Here's how the part is built. I have some questions about the finished solid (model axes, mm). A direction names the side the tool comes from. Round coordinates to 2 decimals unless told otherwise and drop trailing zeros. Write each loop counter-clockwise with the first axis right and the second up, starting at its lowest first coordinate (ties: lowest second). Pieces come first, ordered by that corner, then holes. Notation, with made-up numbers: (-26, 39) - (9, 39) arc R21 ccw to (9, 43) - close; hole circle Ø3 at (45, -18). An arc over 180 degrees is marked (long way). One line per question, with ' | ' between items. Start each with the question number.
(1) For faces 5 (the flat face through (-2, -48.26, 4)), 6 (the flat face through (-2, -50.8, 3)), which set-ups out of +Z, -Z, +X, -X, +Y, -Y let a thin tool reach every point of the face, with its end or its side?
(2) Imagine slicing it at A-A (z = 3.25). Write out the boundary of the cut face in (x, y).
(3) Will these pins go through, and if not, where does the flat tip stop? pin 1 (8 mm diameter, centred on x = -18, y = -9.5, fed in from -Z); pin 2 (10 mm diameter, centred on x = 13.5, y = -35.5, fed in from +Z); pin 3 (2 mm diameter, centred on x = -8, y = -21.5, fed in from +Z).
(4) Imagine slicing it at D-D (z = -6.25). Write out the boundary of the cut face in (x, y).
(5) If I drill on L1, parallel to Y at x = -5.5, z = 9.5; L2, parallel to X at y = -32, z = 3.25; L3, parallel to X at y = -8.5, z = -9, over which ranges is the centre line in solid material (lowest first)?
(6) Thinking about a two-plate mould opening in X: for faces 1 (the flat face through (-2, -2.54, 4)), 2 (the flat face through (0, -50, 12.7)), 3 (the flat face through (-13.842, -25.044, -6.261)), 4 (the flat face through (23.497, -25, 6)), which applies, pulls with the +X half, pulls with the -X half, needs draft (parallel to the pull), parting line crosses it, or undercut?
(7) Imagine slicing it at C-C (x = -5). Write out the boundary of the cut face in (y, z), plus the area to 3 significant figures.
(8) Imagine slicing it at B-B (y = -19). Write out the boundary of the cut face in (x, z).
from build123d import *

# Parameters (mm, degrees)
F1_DEPTH = 50.8
F2_T     = -2.54


with BuildPart() as f1:
    # F0 (on Front) → F1 (new body)
    with BuildSketch(Plane.XZ):
        Polygon((23.497318, 12.7), (0, 12.7), (0, -12.7), (23.497318, 0), align=None)
        Polygon((0, 12.7), (-27.302682, 12.7), (-27.302682, 0), (0, -12.7), align=None)
    extrude(amount=F1_DEPTH)

    # F2
    f2_openings = [f1.faces().sort_by_distance(p)[0] for p in [
        (-1.902682, -25.4, 12.7),
    ]]
    offset(amount=F2_T, openings=f2_openings)


solid = f1.part
Check sheet entries:
1) face 5: +Z | face 6: +Z, -Z, +X, -X, -Y
2) outline: (-27.3, -50.8) - (23.5, -50.8) - (23.5, 0) - (-27.3, 0) - close; hole (-24.76, -48.26) - (20.96, -48.26) - (20.96, -2.54) - (-24.76, -2.54) - close
3) pin 1: z = -6.19 | pin 2: z = 0.19 | pin 3: z = -5.71
4) outline: (-13.87, -50.8) - (11.93, -50.8) - (11.93, 0) - (-13.87, 0) - close; hole (-7.84, -48.26) - (6.59, -48.26) - (6.59, -2.54) - (-7.84, -2.54) - close
5) L1: -50.8 to -48.26, -2.54 to 0 | L2: -27.3 to -24.76, 20.96 to 23.5 | L3: -7.95 to -1.93, 1.5 to 6.85
6) face 1: undercut | face 2: needs draft | face 3: pulls with the -X half | face 4: pulls with the +X half
7) outline: (-50.8, -10.37) - (0, -10.37) - (0, 12.7) - (-2.54, 12.7) - (-2.54, -7.57) - (-48.26, -7.57) - (-48.26, 12.7) - (-50.8, 12.7) - close | area: 245 mm^2
8) outline: (-27.3, 0) - (0, -12.7) - (23.5, 0) - (23.5, 12.7) - (20.96, 12.7) - (20.96, 1.51) - (-0.09, -9.86) - (-24.76, 1.62) - (-24.76, 12.7) - (-27.3, 12.7) - close
